from build123d import *

# Parameters (mm, degrees)
F0_W     = 30
F0_H     = 30
F1_DEPTH = 2
F2_R     = 5
F3_DEPTH = 8
F4_R     = 3
F5_R     = 1.99999


# Not quite as in the source:
# - a fillet or chamfer is up to 0.001 mm smaller than in the source, because OpenCascade refuses the exact size


with BuildPart() as f1:
    # F0 (on Top) → F1 (new body)
    with BuildSketch(Plane.XY):
        Rectangle(F0_W, F0_H)
    extrude(amount=F1_DEPTH)

    # F2 (on face) → F3 (join)
    with BuildSketch(Plane.XY.offset(2)):
        Circle(F2_R)
    extrude(amount=F3_DEPTH)

    # F4
    f4_edges = [f1.edges().sort_by_distance(p)[0] for p in [
        (-5, 0, 10),
    ]]
    fillet(f4_edges, radius=F4_R)

    # F5 (radius 2 in the source; OpenCascade refuses exactly that, so slightly less here)
    f5_edges = [f1.edges().sort_by_distance(p)[0] for p in [
        (0, -15, 2),
        (-15, 0, 2),
        (15, 0, 2),
        (0, 15, 2),
        (-5, 0, 2),
    ]]
    fillet(f5_edges, radius=F5_R)


solid = f1.part
Work out the finished part from the listing and answer in its coordinate system (mm). A direction names the side the tool comes from. Give positions to 0.01 mm unless a question says otherwise; leave off trailing zeros. Use a Markdown table: item, result. Add a question column.
1) Each of these flat-tipped pins is pushed along its axis until it touches: P1, Ø1, axis at y = 6.5, z = 8, coming from the +X side; P2, Ø10, axis at x = 10.5, y = -3, coming from the +Z side; P3, Ø2, axis at x = -9, y = 4.5, coming from the -Z side; P4, Ø6, axis at x = -8.5, y = 11, coming from the +Z side. Where does it stop, or does it pass through?
2) Consider line 1 along Z through (x, y) = (9, 0.75); line 2 along X through (y, z) = (3.5, 4.75); line 3 along Y through (x, z) = (0.5, 5.5). Determine where each line is inside the solid, lowest interval first.
3) Which of the six approach directions +Z, -Z, +X, -X, +Y, -Y give full straight-line access (tool end or side, diameter ignored) to faces 1 (the cylindrical face through (0.21, -14.4, 1.43)), 2 (the cylindrical face through (-1.08, -4.88, 5.48))?
Reported:
| question | item | result |
|---|---|---|
| 1 | P1 | passes through |
| 1 | P2 | stops at z = 2.32 |
| 1 | P3 | stops at z = 0 |
| 1 | P4 | stops at z = 2 |
| 2 | line 1 | z = 0 to 2 |
| 2 | line 2 | x = -3.57 to 3.57 |
| 2 | line 3 | y = -4.97 to 4.97 |
| 3 | face 1 | +Z, +X, -X, -Y |
| 3 | face 2 | +Z |
